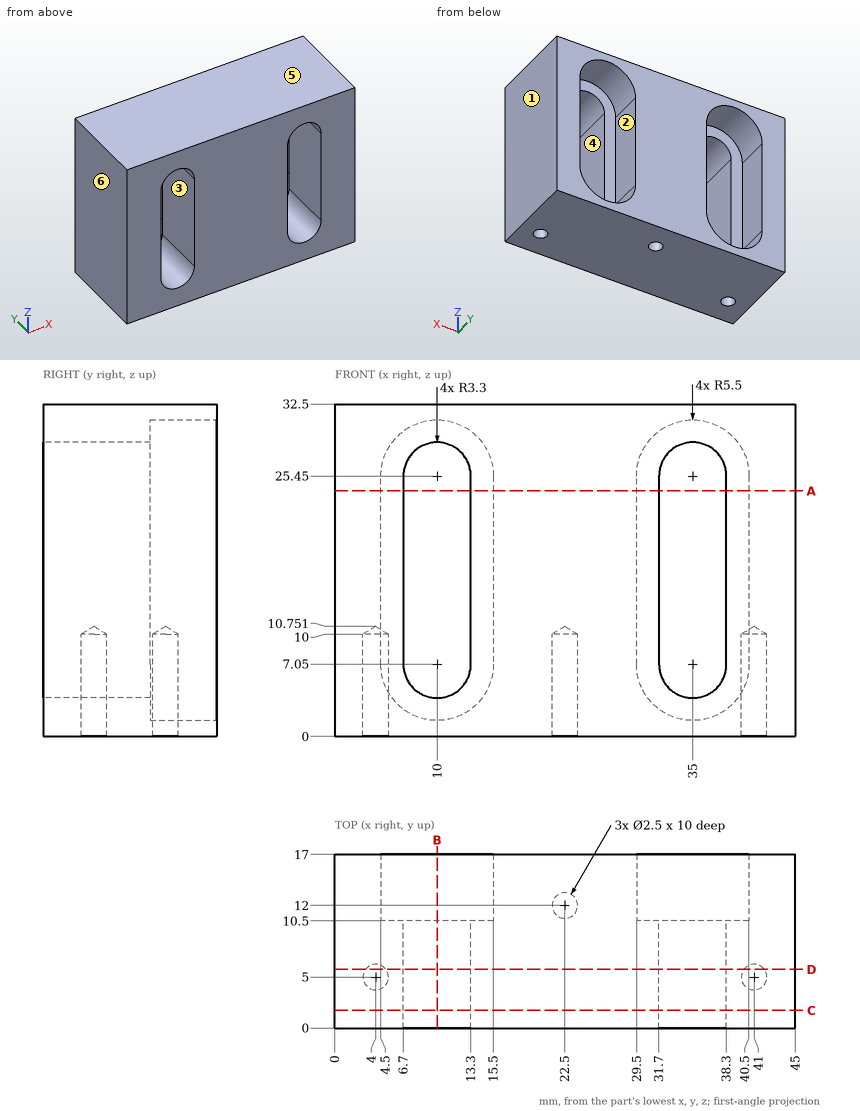
Can you work these out from the drawing? Everything is in mm from the part's minimum corner. A direction names the side the tool comes from. Give positions to 0.01 mm unless a question says otherwise; leave off trailing zeros. Order: outer loops, then holes, each group sorted by start corner. A loop starts at its lowest first (then second) coordinate and runs counter-clockwise, first axis right, second up. Notation, with made-up numbers: M -10,24 L 8,24 A10 cw 8,43 Z; hole C 29,71 d7. An arc over 180 degrees is marked long. Write item = value, one per line. Start each with the question number.
Q1. Suppose I cut it at A-A (z = 24). Write out the boundary of the cut face in (x, y), plus the area to 3 significant figures.
Q2. Suppose I cut it at C-C (y = 1.75). Write out the boundary of the cut face in (x, z).
Q3. I need wall thicknesses on probe 1 along X at (y, z) = (7.75, 15); probe 2 along X at (y, z) = (14, 25); probe 3 along Y at (x, z) = (22.5, 4.25). Which ranges of each line are inside material? Lowest first, please. Write a range as [from, to].
Q4. For the marked faces 1, 2 and 3, which set-ups out of +Z, -Z, +X, -X, +Y, -Y let a thin tool reach every point of the face, with its end or its side?
Q5. Will this pin go through, and if not, where does the flat tip stop? pin 1 Ø1.5 at (x, y) = (41, 5) entering from -Z.
Q6. Suppose I cut it at B-B (x = 10). Write out the boundary of the cut face in (y, z), plus the area to 3 significant figures.
Q7. Suppose I cut it at D-D (y = 5.75). Count the separate pieces of the cut face and the enclosed holes in it, plus the area to 3 significant figures.
Q8. We'd pull the mould along X, two halves only. Please class the marked faces 4, 5 and 6: pulls with the +X half, pulls with the -X half, needs draft (parallel to the pull), parting line crosses it, or undercut.
Check result:
q1.outline = M 0,0 L 6.7,0 L 6.7,10.5 L 4.5,10.5 L 4.5,17 L 0,17 Z; M 13.3,0 L 31.7,0 L 31.7,10.5 L 29.5,10.5 L 29.5,17 L 15.5,17 L 15.5,10.5 L 13.3,10.5 Z; M 38.3,0 L 45,0 L 45,17 L 40.5,17 L 40.5,10.5 L 38.3,10.5 Z
q1.area = 483 mm2
q2.outline = M 0,0 L 45,0 L 45,32.5 L 0,32.5 Z; hole M 6.7,7.05 A3.3 ccw 13.3,7.05 L 13.3,25.45 A3.3 ccw 6.7,25.45 Z; hole M 31.7,7.05 A3.3 ccw 38.3,7.05 L 38.3,25.45 A3.3 ccw 31.7,25.45 Z
q3.probe_1 = [0, 6.7], [13.3, 31.7], [38.3, 45]
q3.probe_2 = [0, 4.5], [15.5, 29.5], [40.5, 45]
q3.probe_3 = [0, 10.75], [13.25, 17]
q4.face_1 = +Z, -Z, +X, +Y, -Y
q4.face_2 = +Y
q4.face_3 = +Y, -Y
q5.pin_1 = 10.3
q6.outline = M 0,0 L 17,0 L 17,1.55 L 10.5,1.55 L 10.5,3.75 L 0,3.75 Z; M 0,28.75 L 10.5,28.75 L 10.5,30.95 L 17,30.95 L 17,32.5 L 0,32.5 Z
q6.area = 98.9 mm2
q7.separate_pieces = 1
q7.enclosed_holes = 2
q7.area = 1,110 mm2
q8.face_4 = undercut
q8.face_5 = needs draft
q8.face_6 = pulls with the -X half
